Autodesk Inventor part; units mm, degrees
ref_plane "YZ Plane" through (0, 0, 0) normal (1, 0, 0) x (0, 1, 0)
ref_plane "XZ Plane" through (0, 0, 0) normal (0, 1, 0) x (-1, 0, 0)
ref_plane "XY Plane" through (0, 0, 0) normal (0, 0, 1) x (1, 0, 0)
sketch "Sketch2" plane through (0, 0, 0) normal (0, 1, 0) x (-1, 0, 0)
  line L0 (0, 0) -> (-15, 0)
  line L1 (-15, 0) -> (-15, 70)
  line L2 (-15, 70) -> (0, 70)
  line L3 (0, 70) -> (0, 0)
  circle A0 centre (-5, 10) radius 2.25
  circle A1 centre (-5, 60) radius 2.25
  circle A2 centre (-7.5, 20) radius 0.95
  circle A3 centre (-7.5, 30) radius 0.95
  circle A4 centre (-7.5, 40) radius 0.95
  circle A5 centre (-7.5, 50) radius 0.95
  dimension "d76" = 15
  dimension "d78" = 10
  dimension "d79" = 50
  dimension "d80" = 5
  dimension "d81" = 4.5
  dimension "d82" = 10
  dimension "d83" = 1.9
  dimension "d86" = 10
  dimension "d91" = 10
  dimension "d92" = 7.5
extrude "Extrusion2" add sketch "Sketch2" along normal blind 6
properties part number "phone_holder_top_insert" material "Acrylic, Clear"
Input: part model. Units: mm. Frame: model coordinates. Coordinates: 2 decimals unless noted, no trailing zeros. Loops run counter-clockwise (first coordinate to the right, second up) from the corner with the lowest first, then second, coordinate; pieces in that order, holes last. Notation, with made-up numbers: M 27,53.25 L 78,53.25 A20 cw 78,78.25 Z; hole C 36.25,41 d6. An arc over 180 degrees is marked long. Use a Markdown table: item, result. Add a question column.
1) Line query: L1, parallel to Z at x = 5, y = 4.2; L2, parallel to Z at x = 7.5, y = 3.25; L3, parallel to Z at x = 6, y = 3.4. Output: solid intervals per line, ascending. Write a range as from..to.
2) Section A-A, the plane z = 40. Return the cut outline in (x, y).
3) Section D-D, the plane z = 10. Return the cut outline in (x, y), plus the area to 3 significant figures.
4) Section C-C, the plane y = 0.95. Return the cut outline in (x, z).
5) Draft query along Z for faces 1 (the cylindrical face through (7.706, 2.958, 50.927)), 2 (the flat face through (0, 3, 35)), 3 (the flat face through (7, 3, 0)). Return one class per face: +Z half, -Z half, draft (parallel to the pull), parting line (faces both ways), or undercut.
6) Section B-B, the plane x = 5. Return the cut outline in (y, z), plus the area to 3 significant figures.
7) Pin query (flat end, axial travel): P1, Ø2, axis at x = 7.5, z = 50, coming from the +Y side. Return the tip coordinate at first contact, or that it passes through.
Answer below:
| question | item | result |
|---|---|---|
| 1 | L1 | 0..7.75, 12.25..57.75, 62.25..70 |
| 1 | L2 | 0..19.05, 20.95..29.05, 30.95..39.05, 40.95..49.05, 50.95..70 |
| 1 | L3 | 0..7.98, 12.02..57.98, 62.02..70 |
| 2 | outline | M 0,0 L 6.55,0 L 6.55,6 L 0,6 Z; M 8.45,0 L 15,0 L 15,6 L 8.45,6 Z |
| 3 | outline | M 0,0 L 2.75,0 L 2.75,6 L 0,6 Z; M 7.25,0 L 15,0 L 15,6 L 7.25,6 Z |
| 3 | area | 63.0 mm2 |
| 4 | outline | M 0,0 L 15,0 L 15,70 L 0,70 Z; hole C 5,10 d4.5; hole C 5,60 d4.5; hole C 7.5,20 d1.9; hole C 7.5,30 d1.9; hole C 7.5,40 d1.9; hole C 7.5,50 d1.9 |
| 5 | face 1 | undercut |
| 5 | face 2 | draft |
| 5 | face 3 | -Z half |
| 6 | outline | M 0,0 L 6,0 L 6,7.75 L 0,7.75 Z; M 0,12.25 L 6,12.25 L 6,57.75 L 0,57.75 Z; M 0,62.25 L 6,62.25 L 6,70 L 0,70 Z |
| 6 | area | 366 mm2 |
| 7 | P1 | y = 6 |
